Geometry: final body of the model. Coordinates: model frame, mm. A direction names the side the tool comes from. Coordinates: 2 decimals unless noted, no trailing zeros. Write each loop counter-clockwise with the first axis right and the second up, starting at its lowest first coordinate (ties: lowest second). Pieces come first, ordered by that corner, then holes. Notation, with made-up numbers: (-27, -19) - (-18, -19) arc R27 cw to (-18, 6) - close; hole circle Ø7 at (66, 81). An arc over 180 degrees is marked (long way). Answer as a JSON object with one key per item and string values. Group by question number.
Item 1: Section A-A on z = 2.5. Return loops of the section in (x, y), and give its area (3 significant figures).
Item 2: First-contact query: pin 1 Ø1.5 at (y, z) = (-2, 8) entering from -X; pin 2 Ø5 at (x, y) = (5.5, -1.5) entering from -Z; pin 3 Ø5 at (x, y) = (-19, -1.5) entering from +Z. Flat tips, straight axial feed; report the tip coordinate or a pass-through.
Item 3: Section B-B on y = 0. Return loops of the section in (x, z), and give its area (3 significant figures).
Item 4: Set-up query: faces 1 (the flat face through (-21, 0, 4)), 2 (the flat face through (16, 0, 4)), 3 (the flat face through (-9.75, 0, 6)). Return all of +Z, -Z, +X, -X, +Y, -Y with unobstructed straight access to the full face (end or side cutting, diameter ignored); none if empty.
Item 5: Mould query, pull axis X, two halves, no side actions, for faces 4 (the cylindrical face through (12.039, 0.07, 16.196)), 5 (the flat face through (0, 0, 18)), 6 (the flat face through (9.75, 0, 6)). Classes: pulls with the +X half, pulls with the -X half, needs draft (parallel to the pull), parting line crosses it, or undercut.
Item 6: Line query: line 1 along Y through (x, z) = (-18.75, 1.9); line 2 along X through (y, z) = (0.75, 2); line 3 along X through (y, z) = (-3.75, 1.75). Output: solid intervals per line, ascending. Write a range as from..to.
Item 7: Section C-C on x = 18.75. Return loops of the section in (y, z), and give its area (3 significant figures).
Item 8: Section D-D on z = 10.75. Return loops of the section in (x, y), and give its area (3 significant figures).
```python
from build123d import *

# Parameters (mm, degrees)
F1_W          = 14
F1_H          = 10
F1_R          = 1.6
F2_DEPTH      = 4
F4_DEPTH      = 5
F4_DEPTH_BACK = 5


with BuildPart() as f2:
    # F1 (on Top) → F2 (new body)
    with BuildSketch(Plane.XY):
        with Locations((-16.75, 0)):
            Rectangle(F1_W, F1_H)
        with Locations((-18.75, 0)):
            Circle(F1_R, mode=Mode.SUBTRACT)
    extrude(amount=F2_DEPTH)



with BuildPart() as f2b:
    # F1 (on Top) → F2, piece 2 (new body)
    with BuildSketch(Plane.XY):
        with Locations((16.75, 0)):
            Rectangle(F1_W, F1_H)
        with Locations((18.75, 0)):
            Circle(F1_R, mode=Mode.SUBTRACT)
    extrude(amount=F2_DEPTH)


with BuildPart() as f2_1:
    add(f2.part)

    add(f2b.part)  # F4 merges F2b
    # F3 (on Front) → F4 (join, two sides)
    with BuildSketch(Plane.XZ) as f4_sk:
        with BuildLine():
            Line((-13.75, 0), (-9.75, 0))
            Line((-9.75, 0), (-9.75, 12))
            ThreePointArc((-9.75, 12), (-9.1642135624, 13.4142135624), (-7.75, 14))
            Line((-7.75, 14), (7.75, 14))
            ThreePointArc((7.75, 14), (9.1642135624, 13.4142135624), (9.75, 12))
            Line((9.75, 12), (9.75, 0))
            Line((9.75, 0), (13.75, 0))
            Line((13.75, 0), (13.75, 12))
            ThreePointArc((13.75, 12), (11.9926406871, 16.2426406871), (7.75, 18))
            Line((7.75, 18), (-7.75, 18))
            ThreePointArc((-7.75, 18), (-11.9926406871, 16.2426406871), (-13.75, 12))
            Line((-13.75, 12), (-13.75, 0))
        make_face()
    extrude(amount=F4_DEPTH)
    extrude(f4_sk.sketch, amount=-F4_DEPTH_BACK)


solid = f2_1.part
```
Checks:
{
 "1": {"outline": "(-23.75, -5) - (-9.75, -5) - (-9.75, 5) - (-23.75, 5) - close; (9.75, -5) - (23.75, -5) - (23.75, 5) - (9.75, 5) - close; hole circle Ø3.2 at (-18.75, 0); hole circle Ø3.2 at (18.75, 0)", "area": "264 mm^2"},
 "2": {"pin 1": "x = -13.75", "pin 2": "z = 13.98", "pin 3": "z = 4"},
 "3": {"outline": "(-23.75, 0) - (-20.35, 0) - (-20.35, 4) - (-23.75, 4) - close; (-17.15, 0) - (-9.75, 0) - (-9.75, 12) arc R2 cw to (-7.75, 14) - (7.75, 14) arc R2 cw to (9.75, 12) - (9.75, 0) - (17.15, 0) - (17.15, 4) - (13.75, 4) - (13.75, 12) arc R6 ccw to (7.75, 18) - (-7.75, 18) arc R6 ccw to (-13.75, 12) - (-13.75, 4) - (-17.15, 4) - close; (20.35, 0) - (23.75, 0) - (23.75, 4) - (20.35, 4) - close", "area": "263 mm^2"},
 "4": {"face 1": "+Z, -X, +Y, -Y", "face 2": "+Z, +X, +Y, -Y", "face 3": "-Z, +Y, -Y"},
 "5": {"face 4": "pulls with the +X half", "face 5": "needs draft", "face 6": "undercut"},
 "6": {"line 1": "-5..-1.6, 1.6..5", "line 2": "-23.75..-20.16, -17.34..-9.75, 9.75..17.34, 20.16..23.75", "line 3": "-23.75..-9.75, 9.75..23.75"},
 "7": {"outline": "(-5, 0) - (-1.6, 0) - (-1.6, 4) - (-5, 4) - close; (1.6, 0) - (5, 0) - (5, 4) - (1.6, 4) - close", "area": "27.2 mm^2"},
 "8": {"outline": "(-13.75, -5) - (-9.75, -5) - (-9.75, 5) - (-13.75, 5) - close; (9.75, -5) - (13.75, -5) - (13.75, 5) - (9.75, 5) - close", "area": "80.0 mm^2"}
}
